```python
from build123d import *

# Parameters (mm, degrees)
SKETCH1_W             = 120
SKETCH1_H             = 35
BOSS_EXTRUDE1_DEPTH   = 6
FILLET1_R             = 6
F_6_0MM_DOWEL_HOLE1_D = 7
SKETCH5_R             = 5.25
CUT_EXTRUDE1_DEPTH    = 1.5
SKETCH6_W             = 55
SKETCH6_H             = 23
CUT_EXTRUDE2_DEPTH    = 64.641574462
BOSS_EXTRUDE4_DEPTH   = 8
CHAMFER1_SIZE         = 5
CHAMFER1_SIZE2        = 1.339745962


with BuildPart() as part:
    # Sketch1 → Boss-Extrude1 (new, symmetric)
    with BuildSketch(Plane(origin=(0, 0, 0), x_dir=(1, 0, 0), z_dir=(0, 1, 0))):
        Rectangle(SKETCH1_W, SKETCH1_H)
    extrude(amount=BOSS_EXTRUDE1_DEPTH, both=True)

    # Fillet1
    fillet1_edges = [part.edges().sort_by_distance(p)[0] for p in [
        (60, 6, 0),
        (60, -6, 0),
    ]]
    fillet(fillet1_edges, radius=FILLET1_R - 0.0001)  # a hair under: the kernel refuses the full size

    # Sketch2 → Cut-Revolve1 (revolve, cut)
    with BuildSketch(Plane.XY):
        with BuildLine():
            Line((-61, 18), (-19, 18))
            ThreePointArc((-19, 18), (-40, 39), (-61, 18))
        make_face()
    revolve(axis=Axis((-61, 18, 0), (1, 0, 0)), mode=Mode.SUBTRACT)

    # Ø6.0mm Dowel Hole1 (through all)
    with Locations(Plane.XY.offset(17.5)):
        with Locations((54, 0)):
            Hole(F_6_0MM_DOWEL_HOLE1_D / 2)

    # Sketch5 → Cut-Extrude1 (cut)
    with BuildSketch(Plane.XZ.offset(6)):
        with Locations(Location((-45.5, 10, 0), (0, 0, 270))):
            Circle(SKETCH5_R)
        with Locations(Location((-45.5, -10, 0), (0, 0, 90))):
            Circle(SKETCH5_R)
    extrude(amount=-CUT_EXTRUDE1_DEPTH, mode=Mode.SUBTRACT)

    # Sketch6 → Cut-Extrude2 (cut, through all)
    with BuildSketch(Plane(origin=(0, 6, 0), x_dir=(1, 0, 0), z_dir=(0, 1, 0))):
        with Locations((12.5, 0)):
            Rectangle(SKETCH6_W, SKETCH6_H)
    extrude(amount=-CUT_EXTRUDE2_DEPTH, mode=Mode.SUBTRACT)

    # Sketch8 → Boss-Extrude4 (add)
    with BuildSketch(Plane(origin=(0, 6, 0), x_dir=(1, 0, 0), z_dir=(0, 1, 0))):
        with BuildLine():
            Line((-34, 17.5), (-29.322921748, 17.5))
            ThreePointArc((-29.322921748, 17.5), (-19.5, 0), (-29.322921748, -17.5))
            Line((-29.322921748, -17.5), (-34, -17.5))
            ThreePointArc((-34, -17.5), (-21.5, 0), (-34, 17.5))
        make_face()
    extrude(amount=BOSS_EXTRUDE4_DEPTH)

    # Chamfer1
    chamfer1_edges = [part.edges().sort_by_distance(p)[0] for p in [
        (-21.5, 14, 0),
    ]]
    chamfer1_side = [part.faces().sort_by_distance(p)[0] for p in [
        (-21.5, 10, 0),
    ]]
    chamfer(chamfer1_edges, length=CHAMFER1_SIZE, length2=CHAMFER1_SIZE2, reference=chamfer1_side[0])


solid = part.part
```
Source: CAD feature listing. Evaluate the final solid. Frame: model axes, mm. A direction names the side the tool comes from. Round coordinates to 2 decimals unless told otherwise and drop trailing zeros. Write each loop counter-clockwise with the first axis right and the second up, starting at its lowest first coordinate (ties: lowest second). Pieces come first, ordered by that corner, then holes. Notation, with made-up numbers: M -9.75,-14 L 35.25,-14 A27 ccw 35.25,2 Z; hole C 39.5,42.5 d5. An arc over 180 degrees is marked long. Answer as a JSON object with one key per item and string values. Group by question number.
(1) Reachability of faces 1 (the flat face through (-46, -4.5, -10)), 2 (the flat face through (-58, 6, 0)), 3 (the flat face through (12, 0, 11.5)) from +Z, -Z, +X, -X, +Y, -Y: full face, straight path, thin tool, end or side. Return the list, or none.
(2) Ray query, line 1 (Y direction, x = 54, z = -4.5); line 2 (X direction, y = 4, z = 1); line 3 (X direction, y = -2.75, z = -6.5). Return the intervals inside material, ascending. Write a range as [from, to].
(3) Mould query, pull axis Z, two halves, no side actions, for faces 4 (the conical face through (-21.121, 10.424, 0.328)), 5 (the cylindrical face through (58.196, 4.289, -0.245)), 6 (the cylindrical face through (-19.502, 9.944, -0.294)). Classes: +Z half, -Z half, draft (parallel to the pull), parting line (faces both ways), or undercut.
(4) Section query C-C on z = 1.5. State how many separate pieces and enclosed holes the cut face has, then the cut area to 3 significant figures.
(5) Section query A-A on y = 2. Output: boundary loops of the cut face in (x, z), then the cut area to 3 significant figures.
(6) Section query D-D on x = -45.5. Output: boundary loops of the cut face in (y, z), then the cut area to 3 significant figures.
(7) First-contact query: pin 1 (9.5 mm diameter, centred on x = -45.5, z = -10, fed in from +Y); pin 2 (6.5 mm diameter, centred on x = -45.5, z = 10, fed in from -Y); pin 3 (6 mm diameter, centred on y = 6.5, z = 7, fed in from +X); pin 4 (12 mm diameter, centred on x = 17, z = 4, fed in from -Y). Flat tips, straight axial feed; report the tip coordinate or a pass-through.
(8) Section query B-B on x = 3. Output: boundary loops of the cut face in (y, z), then the cut area to 3 significant figures.
Computed values:
{
 "1": {"face 1": "-Y", "face 2": "-X, +Y", "face 3": "+Y, -Y"},
 "2": {"line 1": "[-6, -3.5], [3.5, 6]", "line 2": "[-60, -55.62], [-24.38, -15], [40, 58.47]", "line 3": "[-60, -15], [40, 51.83], [56.17, 59.33]"},
 "3": {"face 4": "undercut", "face 5": "draft", "face 6": "parting line"},
 "4": {"separate pieces": "2", "enclosed holes": "1", "area": "523 mm^2"},
 "5": {"outline": "M -60,-17.5 L 51.13,-17.5 L 51.13,17.5 L -60,17.5 Z; M 56.87,-17.5 L 59.66,-17.5 L 59.66,17.5 L 56.87,17.5 Z; hole C -40,0 d27.2; hole M -15,-11.5 L 40,-11.5 L 40,11.5 L -15,11.5 Z", "area": "2,140 mm^2"},
 "6": {"outline": "M -6,-17.5 L 6,-17.5 L 6,-16.33 A20.27 cw 6,16.33 L 6,17.5 L -6,17.5 L -6,15.25 L -4.5,15.25 L -4.5,4.75 L -6,4.75 L -6,-4.75 L -4.5,-4.75 L -4.5,-15.25 L -6,-15.25 Z", "area": "200 mm^2"},
 "7": {"pin 1": "y = 4.59", "pin 2": "y = -4.5", "pin 3": "x = 58.87", "pin 4": "through"},
 "8": {"outline": "M -6,-17.5 L 6,-17.5 L 6,-11.5 L -6,-11.5 Z; M -6,11.5 L 6,11.5 L 6,17.5 L -6,17.5 Z", "area": "144 mm^2"}
}
